Build history of the part. All positions in model axes, mm. A direction names the side the tool comes from. Give positions to 0.01 mm unless a question says otherwise; leave off trailing zeros. Loops run counter-clockwise (first coordinate to the right, second up) from the corner with the lowest first, then second, coordinate; pieces in that order, holes last.
1) Two-plate mould, pull along Y, no slides. Class faces 1 (the flat face through (12.1, -12, -0.4)), 2 (the flat face through (28, -6, 0)), 3 (the cylindrical face through (26.463, -4.226, 1.317)): +Y half, -Y half, draft (parallel to the pull), parting line (faces both ways), or undercut.
2) 3-axis set-ups, long thin cutter, end or side, ignore diameter. For faces 4 (the cylindrical face through (29, -2, 1)), 5 (the flat face through (11, -6, 0)): which of +Z, -Z, +X, -X, +Y, -Y reach the whole face in a straight line?
3) Flat gauge pins, fed straight in: P1, Ø5, axis at x = 24, y = -6.5, coming from the +Z side; P2, Ø3.5, axis at x = 13, y = -3, coming from the +Z side; P3, Ø5, axis at x = 27.5, y = -6.5, coming from the -Z side. Where does each tip first touch, or does it go through?
4) Band-saw the part on A-A on y = -7.5. List the corners of the cut face in (x, z), then the cut area to 3 significant figures.
5) Band-saw the part on D-D on y = -1.25. List the corners of the cut face in (x, z), then the cut area to 3 significant figures.
6) Wall check: line 1 (Y direction, x = 8, z = -1.15); line 2 (Z direction, x = 12, y = -5.75); line 3 (X direction, y = -4, z = 0.6). Give the ranges that are in metal, low to high.
7) Band-saw the part on C-C on x = 3. List the corners of the cut face in (y, z).
```python
from build123d import *

# Parameters (mm, degrees)
F1_DEPTH = 12
F2_R     = 6
F3_R     = 5.99999
F5_D     = 5.25
F5_DEPTH = 12
F5_TIP   = 1.5772591249
F7_D     = 4
F7_DEPTH = 12
F7_TIP   = 1.2017212381


# Not quite as in the source:
# - a fillet or chamfer is up to 0.001 mm smaller than in the source, because OpenCascade refuses the exact size


with BuildPart() as f1:
    # F0 (on Front) → F1 (new body)
    with BuildSketch(Plane.XZ):
        Polygon((17.5538621843, 0), (0, 0), (0, -2.4168363307), (17.5538621843, -2.4168363307), (20.3523058444, 0), (30.528459698, 0), (30.528459698, 2.6712401304), (20.3523058444, 2.6712401304), align=None)
    extrude(amount=F1_DEPTH)

    # F2
    f2_edges = [f1.edges().sort_by_distance(p)[0] for p in [
        (30.52846, 0, 1.33562),
    ]]
    fillet(f2_edges, radius=F2_R)

    # F3 (radius 6 in the source; OpenCascade refuses exactly that, so slightly less here)
    f3_edges = [f1.edges().sort_by_distance(p)[0] for p in [
        (30.52846, -12, 1.33562),
    ]]
    fillet(f3_edges, radius=F3_R)

    # F5
    with Locations(Plane.XY.offset(2.6712401304)):
        with Locations((24.528459698, -6)):
            Hole(F5_D / 2, depth=F5_DEPTH)
            with Locations((0, 0, -(F5_DEPTH + F5_TIP / 2))):  # 118° drill point
                Cone(0, F5_D / 2, F5_TIP, mode=Mode.SUBTRACT)

    # F7
    with Locations(Plane.XY):
        with Locations((8.0127185211, -6)):
            Hole(F7_D / 2, depth=F7_DEPTH)
            with Locations((0, 0, -(F7_DEPTH + F7_TIP / 2))):  # 118° drill point
                Cone(0, F7_D / 2, F7_TIP, mode=Mode.SUBTRACT)


solid = f1.part
```
Findings below:
1. face 1: -Y half
1. face 2: draft
1. face 3: undercut
2. face 4: +Z, -Z, +X, +Y
2. face 5: +Z, -X, +Y, -Y
3. P1: stops at z = 2.67
3. P2: stops at z = 0
3. P3: stops at z = 0
4. outline: (0, -2.42) - (6.69, -2.42) - (6.69, 0) - (0, 0) - close; (9.34, -2.42) - (17.55, -2.42) - (20.35, 0) - (22.37, 0) - (22.37, 2.67) - (20.35, 2.67) - (17.55, 0) - (9.34, 0) - close; (26.68, 0) - (30.34, 0) - (30.34, 2.67) - (26.68, 2.67) - close
4. area: 58.3 mm2
5. outline: (0, -2.42) - (17.55, -2.42) - (20.35, 0) - (28.19, 0) - (28.19, 2.67) - (20.35, 2.67) - (17.55, 0) - (0, 0) - close
5. area: 70.5 mm2
6. line 1: y = -12 to -8, -4 to 0
6. line 2: z = -2.42 to 0
6. line 3: x = 18.18 to 22.83, 26.23 to 30.19
7. outline: (-12, -2.42) - (0, -2.42) - (0, 0) - (-12, 0) - close
